Input: part model. Units: mm. Frame: model coordinates. A direction names the side the tool comes from. Give positions to 0.01 mm unless a question says otherwise; leave off trailing zeros. Loops run counter-clockwise (first coordinate to the right, second up) from the corner with the lowest first, then second, coordinate; pieces in that order, holes last. Notation, with made-up numbers: M 23,-15 L 57,-15 A33 ccw 57,23 Z; hole C -1.5,-20 d4. An arc over 180 degrees is marked long. Return JSON: item names as keys, results as strings. Group by question number.
```python
from build123d import *

# Parameters (mm, degrees)
F0_R      = 19.685
F0_R_2    = 10.16
F0_R_3    = 8.89
F1_DEPTH  = 24.892
F2_R      = 19.685
F2_R_2    = 3.175
F3_DEPTH  = 8.382
F4_R      = 9.271
F5_DEPTH  = 8.89
F6_R      = 3.175
F7_DEPTH  = 5.08
F8_R      = 1.778
F9_DEPTH  = 7.747
F10_R     = 2.54
F11_DEPTH = 2.54
F12_R     = 19.05
F12_R_2   = 10.16
F13_DEPTH = 12.7


with BuildPart() as f1:
    # F0 (on Front) → F1 (new body)
    with BuildSketch(Plane.XZ):
        with Locations((-28.321002, 34.417)):
            Circle(F0_R)
        with Locations((-28.321002, 34.417)):
            Circle(F0_R_2, mode=Mode.SUBTRACT)
        with Locations((-28.321002, 34.417)):
            Circle(F0_R_2)
        with Locations((-28.321002, 34.417)):
            Circle(F0_R_3, mode=Mode.SUBTRACT)
        with Locations((-28.321002, 34.417)):
            Circle(F0_R_3)
    extrude(amount=F1_DEPTH)

    # F2 (on face) → F3 (cut)
    with BuildSketch(Plane(origin=(0, 0, 0), x_dir=(-1, 0, 0), z_dir=(0, 1, 0))):
        with Locations((28.321002, 34.417)):
            Circle(F2_R)
        with Locations((28.321002, 34.417)):
            Circle(F2_R_2, mode=Mode.SUBTRACT)
    extrude(amount=-F3_DEPTH, mode=Mode.SUBTRACT)

    # F4 (on face) → F5 (cut)
    with BuildSketch(Plane.XZ.offset(24.892)):
        with Locations((-28.321002, 34.417)):
            Circle(F4_R)
    extrude(amount=-F5_DEPTH, mode=Mode.SUBTRACT)

    # F6 (on face) → F7 (join)
    with BuildSketch(Plane.XZ.offset(16.002)):
        with Locations((-28.321002, 34.417)):
            Circle(F6_R)
    extrude(amount=F7_DEPTH)

    # F8 (on face) → F9 (cut)
    with BuildSketch(Plane.XZ.offset(16.002)):
        with Locations((-32.749631, 38.955461)):
            Circle(F8_R)
        with Locations((-28.243339, 40.75769)):
            Circle(F8_R)
        with Locations((-23.782541, 38.845629)):
            Circle(F8_R)
        with Locations((-21.980312, 34.339337)):
            Circle(F8_R)
        with Locations((-23.892373, 29.878539)):
            Circle(F8_R)
        with Locations((-28.398665, 28.07631)):
            Circle(F8_R)
        with Locations((-32.859463, 29.988371)):
            Circle(F8_R)
        with Locations((-34.661692, 34.494663)):
            Circle(F8_R)
    extrude(amount=-F9_DEPTH, mode=Mode.SUBTRACT)

    # F10 (on face) → F11 (join)
    with BuildSketch(Plane.XZ.offset(21.082)):
        with Locations((-28.321002, 34.417)):
            Circle(F10_R)
    extrude(amount=F11_DEPTH)

    # F12 (on face) → F13 (cut)
    with BuildSketch(Plane(origin=(0, -8.382, 0), x_dir=(-1, 0, 0), z_dir=(0, 1, 0))):
        with Locations((28.321002, 34.417)):
            Circle(F12_R)
        with Locations((28.321002, 34.417)):
            Circle(F12_R_2, mode=Mode.SUBTRACT)
    extrude(amount=-F13_DEPTH, mode=Mode.SUBTRACT)


solid = f1.part
```
Item 1: First-contact query: pin 1 Ø12 at (x, y) = (-26.5, -6.5) entering from -Z; pin 2 Ø4 at (x, z) = (-21.98, 34.34) entering from -Y; pin 3 Ø21.5 at (x, z) = (-28.32, 34.42) entering from -Y; pin 4 Ø3 at (x, z) = (-28.24, 40.76) entering from +Y. Flat tips, straight axial feed; report the tip coordinate or a pass-through.
Item 2: Section A-A, the plane y = -15.5. Give the number of separate pieces and of enclosed holes in the cut face, then the cut area to 3 significant figures.
Item 3: Pull-direction query (X, two-part tool) for faces 1 (the face through (-18, -8.382, 51)), 2 (the face through (-23.29, -12.25, 35.54)), 3 (the face through (-9.545, -16.521, 40.33)); classes: pulls with the +X half, pulls with the -X half, needs draft (parallel to the pull), parting line crosses it, or undercut.
Item 4: Section B-B, the plane x = -21.5. Return loops of the section in (y, z), then the cut area to 3 significant figures.
Item 5: Material intervals for line 1 (Z direction, x = -37, y = -10); line 2 (X direction, y = -15, z = 27.5); line 3 (Y direction, x = -21.5, z = 41), sorted ascending. Write a range as from..to.
Item 6: Reachability of faces 4 (the face through (-27, -21.082, 37)), 5 (the face through (-37.71, -14.64, 30.53)), 6 (the face through (-31.79, -12.25, 40.45)) from +Z, -Z, +X, -X, +Y, -Y: full face, straight path, thin tool, end or side. Return the list, or none.
Item 7: Section C-C, the plane z = 42. Return loops of the section in (x, y).
Item 8: Section D-D, the plane x = -13. Return loops of the section in (y, z).
Answer below:
{
 "1": {"pin 1": "z = 14.73", "pin 2": "y = -16", "pin 3": "y = -24.89", "pin 4": "through"},
 "2": {"separate pieces": "2", "enclosed holes": "9", "area": "322 mm^2"},
 "3": {"face 1": "needs draft", "face 2": "undercut", "face 3": "parting line crosses it"},
 "4": {"outline": "M -24.89,15.95 L -8.38,15.95 L -8.38,16.63 L -21.08,16.63 L -21.08,26.89 L -8.38,26.89 L -8.38,32.63 L -16,32.63 L -16,28.14 L -24.89,28.14 Z; M -24.89,40.7 L -16,40.7 L -16,36.05 L -8.38,36.05 L -8.38,41.95 L -21.08,41.95 L -21.08,52.2 L -8.38,52.2 L -8.38,52.88 L -24.89,52.88 Z", "area": "211 mm^2"},
 "5": {"line 1": "16.75..17.46, 29.13..39.7, 51.38..52.09", "line 2": "-46.75..-46.07, -35.76..-30.08, -26.72..-20.88, -10.57..-9.89", "line 3": "-24.89..-8.38"},
 "6": {"face 4": "-Y", "face 5": "+Y", "face 6": "+Y, -Y"},
 "7": {"outline": "M -46.49,-24.89 L -33.65,-24.89 L -33.65,-16 L -29.52,-16 L -29.52,-8.38 L -35.08,-8.38 L -35.08,-21.08 L -45.8,-21.08 L -45.8,-8.38 L -46.49,-8.38 Z; M -26.97,-16 L -22.99,-16 L -22.99,-24.89 L -10.16,-24.89 L -10.16,-8.38 L -10.85,-8.38 L -10.85,-21.08 L -21.56,-21.08 L -21.56,-8.38 L -26.97,-8.38 Z"},
 "8": {"outline": "M -24.89,22.06 L -8.38,22.06 L -8.38,23.1 L -21.08,23.1 L -21.08,45.74 L -8.38,45.74 L -8.38,46.78 L -24.89,46.78 Z"}
}
